```python
from build123d import *

# Parameters (mm, degrees)
SKETCH3_R           = 1.25
SKETCH3_R_2         = 5.875
BOSS_EXTRUDE2_DEPTH = 3


with BuildPart() as part:
    # Sketch3 → Boss-Extrude2 (new body)
    with BuildSketch(Plane(origin=(0, 0, 0), x_dir=(0, 0, -1), z_dir=(1, 0, 0))):
        with BuildLine():
            Line((-24.261559398, 11.266731363), (-35.997048204, -14.004241165))
            ThreePointArc((-35.997048204, -14.004241165), (-34.876919869, -30.789396433), (-20.125, -38.875))
            Line((-20.125, -38.875), (-15.125, -38.875))
            ThreePointArc((-15.125, -38.875), (-10.004093471, -38.108986863), (-5.33149342, -35.87800758))
            Line((-5.33149342, -35.87800758), (2.552389063, -30.554225285))
            ThreePointArc((2.552389063, -30.554225285), (3.174199215, -30.274562996), (3.853820115, -30.220025911))
            ThreePointArc((3.853820115, -30.220025911), (5.64328781, -29.760501772), (6.738132443, -28.272324263))
            ThreePointArc((6.738132443, -28.272324263), (7.042647171, -27.662299968), (7.534383085, -27.190013348))
            Line((7.534383085, -27.190013348), (14.970074344, -22.168883015))
            ThreePointArc((14.970074344, -22.168883015), (17.351311214, 20.359137977), (-24.261559398, 11.266731363))
        make_face()
        with BuildLine():
            Line((-20.125, -14.875), (-15.125, -14.875))
            ThreePointArc((-15.125, -14.875), (-8.625, -21.375), (-15.125, -27.875))
            Line((-15.125, -27.875), (-20.125, -27.875))
            ThreePointArc((-20.125, -27.875), (-26.625, -21.375), (-20.125, -14.875))
        make_face(mode=Mode.SUBTRACT)
        with BuildLine():
            Line((-22.679384039, -12.875), (-27.679384039, -12.875))
            ThreePointArc((-27.679384039, -12.875), (-29.304384039, -11.25), (-27.679384039, -9.625))
            Line((-27.679384039, -9.625), (-22.679384039, -9.625))
            ThreePointArc((-22.679384039, -9.625), (-21.054384039, -11.25), (-22.679384039, -12.875))
        make_face(mode=Mode.SUBTRACT)
        with Locations((4.104308205, -27.481457724)):
            Circle(SKETCH3_R, mode=Mode.SUBTRACT)
        with Locations((6.277610864, -16.958330561)):
            Circle(SKETCH3_R, mode=Mode.SUBTRACT)
        with Locations((20.80047509, -9.625)):
            Circle(SKETCH3_R, mode=Mode.SUBTRACT)
        with Locations((-10.322617138, 0)):
            Circle(SKETCH3_R, mode=Mode.SUBTRACT)
        Circle(SKETCH3_R_2, mode=Mode.SUBTRACT)
        with Locations((9.189505152, 4.140062296)):
            Circle(SKETCH3_R, mode=Mode.SUBTRACT)
        with BuildLine():
            Line((-7.570615961, -33.125), (-12.570615961, -33.125))
            ThreePointArc((-12.570615961, -33.125), (-14.195615961, -31.5), (-12.570615961, -29.875))
            Line((-12.570615961, -29.875), (-7.570615961, -29.875))
            ThreePointArc((-7.570615961, -29.875), (-5.945615961, -31.5), (-7.570615961, -33.125))
        make_face(mode=Mode.SUBTRACT)
        with Locations((-28.41801633, -3.655785684)):
            Circle(SKETCH3_R, mode=Mode.SUBTRACT)
    extrude(amount=BOSS_EXTRUDE2_DEPTH)


solid = part.part
```
The model under review builds one solid part; all positions refer to its coordinate system, in mm. A direction names the side the tool comes from. Give positions to 0.01 mm unless a question says otherwise; leave off trailing zeros. Write each loop counter-clockwise with the first axis right and the second up, starting at its lowest first coordinate (ties: lowest second). Pieces come first, ordered by that corner, then holes. Notation, with made-up numbers: (-4.75, 12.5) - (38.25, 12.5) arc R26 ccw to (38.25, 37.5) - close; hole circle Ø6 at (26.5, 64.25). An arc over 180 degrees is marked (long way). Answer in a Markdown table with one row per item. Add a question column.
1. Wall thickness on line 1 along Z through (x, y) = (2.8, 4); line 2 along Y through (x, z) = (2.2, -4); line 3 along Z through (x, y) = (2.2, 0.5): over which ranges is each line inside the solid? List them lowest first. Write a range as [from, to].
2. We need section B-B on z = 0. Write out the cut boundary in (x, y) (3 decimals), then the cut area to 3 significant figures.
3. We need section D-D on x = 2.35. State how many separate pieces and enclosed holes the cut face has, then the cut area to 3 significant figures.
4. Tool access review of faces 1 (the cylindrical face through (1.479, -21.232, 8.627)), 2 (the flat face through (1.479, -1.192, 30.047)): name each direction out of +Z, -Z, +X, -X, +Y, -Y from which nothing blocks a thin tool from reaching the whole face with its end or side.
5. We need section A-A on y = -31.5. Write out the cut boundary in (x, z), then the cut area to 3 significant figures.
6. Draft analysis for pull direction Y (two halves, no side actions). For faces 3 (the flat face through (0, -6, 6)), 4 (the cylindrical face through (1.479, -21.518, 26.623)), 5 (the flat face through (1.479, -24.715, -11.2)), state which applies: +Y half, -Y half, draft (parallel to the pull), parting line (faces both ways), or undercut.
7. We need section C-C on y = 0. Write out the cut boundary in (x, z) (3 decimals), then the cut area to 3 significant figures.
8. Insertion check: P1, Ø2, axis at y = -9.62, z = -20.8, coming from the +X side; P2, Ø1, axis at x = 2, y = 4, coming from the -Z side; P3, Ø1.5, axis at x = 1.5, z = 10, coming from the +Y side; P4, Ø1, axis at x = 0.5, y = 1, coming from the -Z side. Each pin has a flat end and moves straight along its axis. Give the tip position at first contact, or say it passes through.
Ans:
| question | item | result |
|---|---|---|
| 1 | line 1 | z = [-26.45, -10.43], [-7.95, -4.3], [4.3, 27.64] |
| 1 | line 2 | y = [-30.23, -28.73], [-26.24, -4.3], [4.3, 26.45] |
| 1 | line 3 | z = [-26.75, -5.85], [5.85, 9.18], [11.47, 29.26] |
| 2 | outline | (0, -32.278) - (3, -32.278) - (3, -5.875) - (0, -5.875) - close; (0, 5.875) - (3, 5.875) - (3, 26.75) - (0, 26.75) - close |
| 2 | area | 142 mm^2 |
| 3 | separate pieces | 1 |
| 3 | enclosed holes | 10 |
| 3 | area | 2,630 mm^2 |
| 4 | face 1 | +X, -X |
| 4 | face 2 | +Z, +X, -X, +Y |
| 5 | outline | (0, -1.15) - (3, -1.15) - (3, 5.95) - (0, 5.95) - close; (0, 14.2) - (3, 14.2) - (3, 34.4) - (0, 34.4) - close |
| 5 | area | 81.9 mm^2 |
| 6 | face 3 | draft |
| 6 | face 4 | undercut |
| 6 | face 5 | -Y half |
| 7 | outline | (0, -26.75) - (3, -26.75) - (3, -5.875) - (0, -5.875) - close; (0, 5.875) - (3, 5.875) - (3, 9.073) - (0, 9.073) - close; (0, 11.573) - (3, 11.573) - (3, 29.494) - (0, 29.494) - close |
| 7 | area | 126 mm^2 |
| 8 | P1 | passes through |
| 8 | P2 | stops at z = -26.52 |
| 8 | P3 | stops at y = 25.1 |
| 8 | P4 | stops at z = -26.75 |
